Check sheet for the drawn part. Datum: minimum x, y, z corner. Units: mm. A direction names the side the tool comes from. Give positions to 0.01 mm unless a question says otherwise; leave off trailing zeros. Order: outer loops, then holes, each group sorted by start corner. A loop starts at its lowest first (then second) coordinate and runs counter-clockwise, first axis right, second up. Notation, with made-up numbers: M 26,34.25 L 39,34.25 A34 cw 39,66.25 Z; hole C 52,28.25 d3. An arc over 180 degrees is marked long. Answer as CSV lines item,"result". Start each with the question number.
Q1. Go/stop test with flat-tipped pins: pin 1 (3.5 mm diameter, centred on x = 15.5, y = 2, fed in from -Z) (3 decimals); pin 2 (2 mm diameter, centred on y = 2.5, z = 24.5, fed in from -X). Record where each tip stops, or that it passes through.
Q2. Section check B-B, the plane y = 3.5. Record the boundary of the cut face in (x, z) (3 decimals), then the cut area to 4 significant figures.
Q3. Thickness scan on line 1 (X direction, y = 5.75, z = 22); line 2 (Z direction, x = 21.75, y = 4) (3 decimals). Record the ranges inside material, lowest first.
Q4. Section check A-A, the plane z = 16.5. Record the boundary of the cut face in (x, y).
Q5. Section check C-C, the plane x = 17.25. Record the boundary of the cut face in (y, z) (3 decimals).
Q6. Set-up check for the marked faces 1 and 2: record each of +Z, -Z, +X, -X, +Y, -Y from which the full face is reachable in a straight line by a thin tool's end or side.
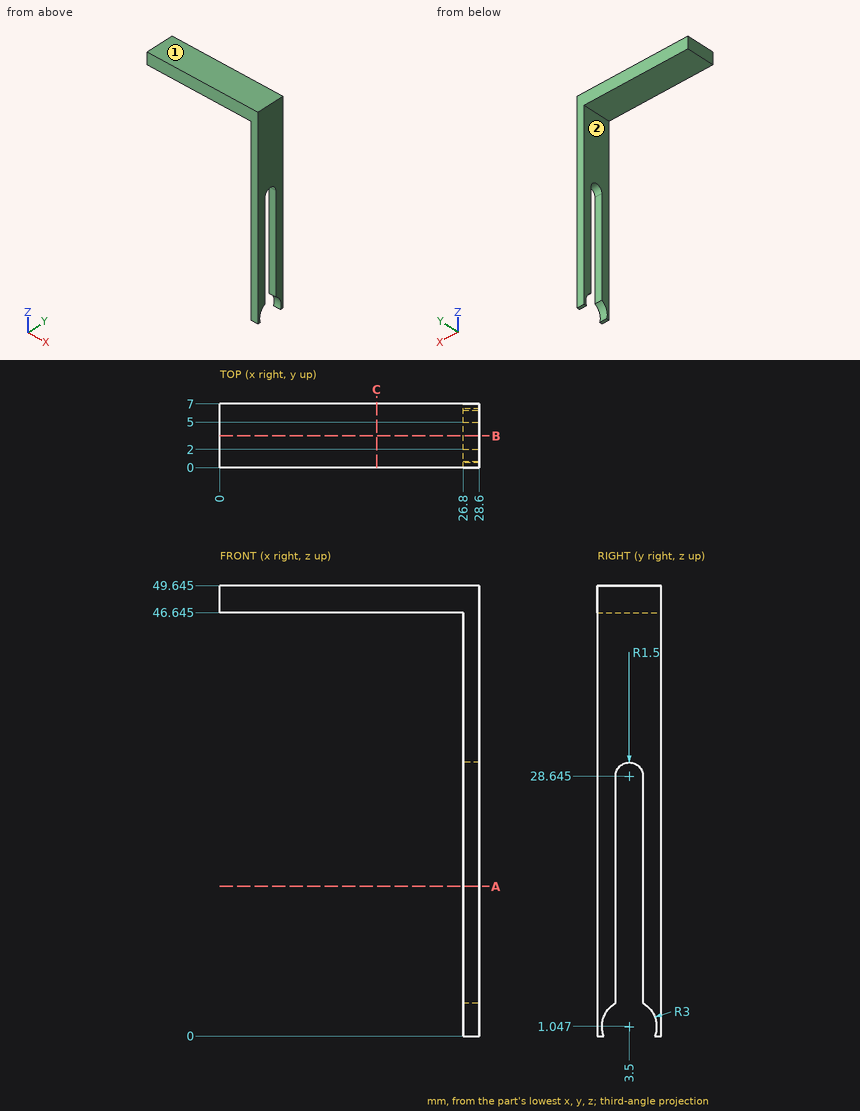
Answer block:
1,pin 1,"stops at z = 46.645"
1,pin 2,"stops at x = 26.8"
2,outline,"M 0,46.645 L 26.8,46.645 L 26.8,30.145 L 28.6,30.145 L 28.6,49.645 L 0,49.645 Z"
2,area,"115.5 mm2"
3,line 1,"x = 26.8 to 28.6"
3,line 2,"z = 46.645 to 49.645"
4,outline,"M 26.8,0 L 28.6,0 L 28.6,2 L 26.8,2 Z; M 26.8,5 L 28.6,5 L 28.6,7 L 26.8,7 Z"
5,outline,"M 0,46.645 L 7,46.645 L 7,49.645 L 0,49.645 Z"
6,face 1,"+Z, +X, -X, +Y, -Y"
6,face 2,"-Z, -X, +Y, -Y"
